from build123d import *

# Parameters (mm, degrees)
SKETCH1_R           = 3.5
BOSS_EXTRUDE1_DEPTH = 6.8
SKETCH2_W           = 15
SKETCH2_H           = 7
CUT_EXTRUDE1_DEPTH  = 6.8
SKETCH3_R           = 2.75
CUT_EXTRUDE2_DEPTH  = 6.8
CIRPATTERN1_COUNT   = 3
CUT_EXTRUDE3_DEPTH  = 6.8
FILLET1_R           = 13


with BuildPart() as part:
    # Sketch1 → Boss-Extrude1 (new body)
    with BuildSketch(Plane.XY):
        with BuildLine():
            Line((-96.50625, -185), (96.50625, -185))
            ThreePointArc((96.50625, -185), (191.056759621, -110.306671598), (208.4678247, 8.923135876))
            Line((208.4678247, 8.923135876), (111.9615747, 176.076864124))
            ThreePointArc((111.9615747, 176.076864124), (0, 220.613343196), (-111.9615747, 176.076864124))
            Line((-111.9615747, 176.076864124), (-208.4678247, 8.923135876))
            ThreePointArc((-208.4678247, 8.923135876), (-191.056759621, -110.306671598), (-96.50625, -185))
        make_face()
        Circle(SKETCH1_R, mode=Mode.SUBTRACT)
    extrude(amount=BOSS_EXTRUDE1_DEPTH)

    # Sketch2 → Cut-Extrude1 (cut)
    with BuildSketch(Plane.XY.offset(6.8)):
        with Locations((0, -177.5)):
            Rectangle(SKETCH2_W, SKETCH2_H)
        with Locations((71.5, -177.5)):
            Rectangle(SKETCH2_W, SKETCH2_H)
        with Locations((-71.5, -177.5)):
            Rectangle(SKETCH2_W, SKETCH2_H)
    cut_extrude1 = extrude(amount=-CUT_EXTRUDE1_DEPTH, mode=Mode.SUBTRACT)

    # Sketch3 → Cut-Extrude2 (cut)
    with BuildSketch(Plane.XY.offset(6.8)):
        with Locations((0, 195.5)):
            Circle(SKETCH3_R)
    cut_extrude2 = extrude(amount=-CUT_EXTRUDE2_DEPTH, mode=Mode.SUBTRACT)

    # CirPattern1: Cut-Extrude1, Cut-Extrude2 ×3 about axis
    cirpattern1_axis = Axis((0, 0, 0), (0, 0, 1))
    for i in range(1, CIRPATTERN1_COUNT):
        add(cut_extrude1.rotate(cirpattern1_axis, i * 360 / CIRPATTERN1_COUNT), mode=Mode.SUBTRACT)
        add(cut_extrude2.rotate(cirpattern1_axis, i * 360 / CIRPATTERN1_COUNT), mode=Mode.SUBTRACT)

    # Sketch4 → Cut-Extrude3 (cut)
    with BuildSketch(Plane.XY.offset(6.8)):
        Polygon((-117.162140817, 123.069219382), (-165.162140817, 39.930780618), (-39.588457268, -32.569219382), (8.411542732, 50.569219382), align=None)
    extrude(amount=-CUT_EXTRUDE3_DEPTH, mode=Mode.SUBTRACT)

    # Fillet1
    fillet1_edges = [part.edges().sort_by_distance(p)[0] for p in [
        (-117.162140817, 123.069219382, 3.4),
        (8.411542732, 50.569219382, 3.4),
        (-39.588457268, -32.569219382, 3.4),
        (-165.162140817, 39.930780618, 3.4),
    ]]
    fillet(fillet1_edges, radius=FILLET1_R)


solid = part.part
Read the model definition and answer for the solid it produces. Units are mm, in the model's axes. A direction names the side the tool comes from. Coordinates: 2 decimals unless noted, no trailing zeros. Loops run counter-clockwise (first coordinate to the right, second up) from the corner with the lowest first, then second, coordinate; pieces in that order, holes last.
Q1. The part is cut by section B-B on x = -26.5. Write down the section's boundary in (y, z).
Q2. Which of the six approach directions +Z, -Z, +X, -X, +Y, -Y give full straight-line access (tool end or side, diameter ignored) to faces 4 (the face through (160.89, 91.33, 3.35)), 5 (the face through (-103.1, 4.1, 3.4))?
Q3. The part is cut by section D-D on y = -133.5. Write down the section's boundary in (x, z), and give its area (3 significant figures).
Q4. The part is cut by section C-C on z = 3.75. Give the number of separate pieces and of enclosed holes in the cut face, and give its area (3 significant figures).
Q5. The mould has two halves that part along X. Classify faces 1 (the face through (-3, -24, 0)), 2 (the face through (-191.91, -108.81, 3.35)), 3 (the face through (-15.83, 8.58, 3.45)): +X half, -X half, draft (parallel to the pull), parting line (faces both ways), or undercut.
Q6. Each of these flat-tipped pins is pushed along its axis until it touches: pin 1 Ø2 at (y, z) = (-179, 2) entering from +X; pin 2 Ø3.5 at (y, z) = (-176.5, 3) entering from -X; pin 3 Ø2 at (y, z) = (-176, 4.5) entering from +X. Where does it stop, or does it pass through?
Q7. The part is cut by section A-A on y = -12. Write down the section's boundary in (x, z).
Q8. Consider probe 1 along Y at (x, z) = (4.5, 6.75); probe 2 along Y at (x, z) = (0, 5); probe 3 along X at (y, z) = (23.5, 6). Determine where each line is inside the solid, lowest interval first.
Results below:
1. outline: (-185, 0) - (-9.9, 0) - (-9.9, 6.8) - (-185, 6.8) - close; (70.73, 0) - (218.44, 0) - (218.44, 6.8) - (70.73, 6.8) - close
2. face 4: +Z, -Z, +X, +Y
2. face 5: +Z, -Z
3. outline: (-174.83, 0) - (174.83, 0) - (174.83, 6.8) - (-174.83, 6.8) - close
3. area: 2,380 mm2
4. separate pieces: 1
4. enclosed holes: 14
4. area: 118,000 mm2
5. face 1: draft
5. face 2: -X half
5. face 3: undercut
6. pin 1: stops at x = 115.55
6. pin 2: stops at x = -122.49
6. pin 3: stops at x = 121.98
7. outline: (-212.03, 0) - (-75.22, 0) - (-75.22, 6.8) - (-212.03, 6.8) - close; (-27.71, 0) - (212.03, 0) - (212.03, 6.8) - (-27.71, 6.8) - close
8. probe 1: y = -185 to -181, -174 to 220.55
8. probe 2: y = -185 to -181, -174 to -3.5, 3.5 to 36, 54.85 to 192.75, 198.25 to 220.61
8. probe 3: x = -200.05 to -195.43, -187.35 to -136.7, -7.22 to 187.35, 195.43 to 200.05
